Source: CAD feature listing. Evaluate the final solid. Frame: model axes, mm. Face numbers are marked on the shaded views. A direction names the side the tool comes from. Coordinates: 2 decimals unless noted, no trailing zeros. Write each loop counter-clockwise with the first axis right and the second up, starting at its lowest first coordinate (ties: lowest second). Pieces come first, ordered by that corner, then holes. Notation, with made-up numbers: (-33.75, 37) -> (-24.75, 37) arc R6 cw to (-24.75, 48) -> close; hole circle Ø10 at (54.25, -8.5). An arc over 180 degrees is marked (long way). One line per item, written item: value. Start each with the question number.
1. Access query for the marked faces 1, 2 and 3. Directions: +Z, -Z, +X, -X, +Y, -Y. A direction counts if a zero-diameter tool reaches every point of the face in a straight line with its end or side. Return the directions, or none.
2. Section query A-A, the plane z = -38. Output: boundary loops of the cut face in (x, y).
3. Mould query, pull axis X, two halves, no side actions, for the marked faces 4, 5 and 6. Classes: released by +X, released by -X, zero draft, split by the parting line, or undercut.
4. Section query C-C, the plane x = -18.5. Output: boundary loops of the cut face in (y, z).
5. First-contact query: P1, Ø1.8, axis at x = -19, y = -1, coming from the +Z side. Flat tip, straight axial feed; report the tip coordinate or a pass-through.
6. Section query B-B, the plane y = -5. Output: boundary loops of the cut face in (x, z).
7. Line query: line 1 (X direction, y = -1, z = -4); line 2 (X direction, y = -0.25, z = -26); line 3 (X direction, y = 0, z = -25). Output: solid intervals per line, ascending.
8. Section query D-D, the plane z = -5.5. Output: boundary loops of the cut face in (x, y), and give its area (3 significant figures).
from build123d import *

# Parameters (mm, degrees)
SALIENTE_EXTRUIR1_DEPTH = 39
CROQUIS2_W              = 8.25
CROQUIS2_H              = 28
CROQUIS2_W_2            = 1.05
CORTAR_EXTRUIR1_DEPTH   = 7
SALIENTE_EXTRUIR4_DEPTH = 3
SALIENTE_EXTRUIR5_DEPTH = 3
CROQUIS4_R              = 2.1
CORTAR_EXTRUIR2_DEPTH   = 52.548520832


with BuildPart() as part:
    # Croquis1 → Saliente-Extruir1 (new body)
    with BuildSketch(Plane.XY):
        with BuildLine():
            Line((-22.1, 1), (-28.5, 1))
            Line((-28.5, 1), (-28.5, -8))
            Line((-28.5, -8), (28.5, -8))
            Line((28.5, -8), (28.5, 1))
            Line((28.5, 1), (20.2, 1))
            ThreePointArc((20.2, 1), (15.5, -3.7), (10.8, 1))
            Line((10.8, 1), (1.2, 1))
            ThreePointArc((1.2, 1), (-3.5, -3.7), (-8.2, 1))
            Line((-8.2, 1), (-14.9, 1))
            ThreePointArc((-14.9, 1), (-18.5, -2.6), (-22.1, 1))
        make_face()
    extrude(amount=-SALIENTE_EXTRUIR1_DEPTH)

    # Croquis2 → Cortar-Extruir1 (cut)
    with BuildSketch(Plane(origin=(0, 1, 0), x_dir=(1, 0, 0), z_dir=(0, 1, 0))):
        with Locations((-19.025, 17.5)):
            Rectangle(CROQUIS2_W, CROQUIS2_H)
        with Locations((-14.375, 17.5)):
            Rectangle(CROQUIS2_W_2, CROQUIS2_H)
    extrude(amount=-CORTAR_EXTRUIR1_DEPTH, mode=Mode.SUBTRACT)

    # Croquis3 → Saliente-Extruir4 (add)
    with BuildSketch(Plane(origin=(0, 0, -39), x_dir=(-1, 0, 0), z_dir=(0, 0, -1))):
        with BuildLine():
            Line((-28.5, 1), (-28.5, -8))
            Line((-28.5, -8), (13.5, -8))
            Line((13.5, -8), (13.5, 1))
            Line((13.5, 1), (5, 1))
            ThreePointArc((5, 1), (3.5, -0.5), (2, 1))
            Line((2, 1), (-14, 1))
            ThreePointArc((-14, 1), (-15.5, -0.5), (-17, 1))
            Line((-17, 1), (-28.5, 1))
        make_face()
    extrude(amount=SALIENTE_EXTRUIR4_DEPTH)

    # Croquis3_4 → Saliente-Extruir5 (add, symmetric)
    with BuildSketch(Plane(origin=(0, 0, -39), x_dir=(-1, 0, 0), z_dir=(0, 0, -1))):
        with BuildLine():
            Line((13.5, 1), (13.5, -8))
            Line((13.5, -8), (28.5, -8))
            Line((28.5, -8), (28.5, 1))
            Line((28.5, 1), (20.5, 1))
            ThreePointArc((20.5, 1), (18.5, -1), (16.5, 1))
            Line((16.5, 1), (13.5, 1))
        make_face()
    extrude(amount=SALIENTE_EXTRUIR5_DEPTH, both=True)

    # Croquis4 → Cortar-Extruir2 (cut, through all)
    with BuildSketch(Plane(origin=(0, 1, 0), x_dir=(1, 0, 0), z_dir=(0, 1, 0))):
        with Locations(Location((-24.5, 38, 0), (0, 0, 270))):
            Circle(CROQUIS4_R)
        with Locations(Location((24.5, 38, 0), (0, 0, 270))):
            Circle(CROQUIS4_R)
        with Locations(Location((24.5, 4, 0), (0, 0, 270))):
            Circle(CROQUIS4_R)
    extrude(amount=-CORTAR_EXTRUIR2_DEPTH, mode=Mode.SUBTRACT)


solid = part.part
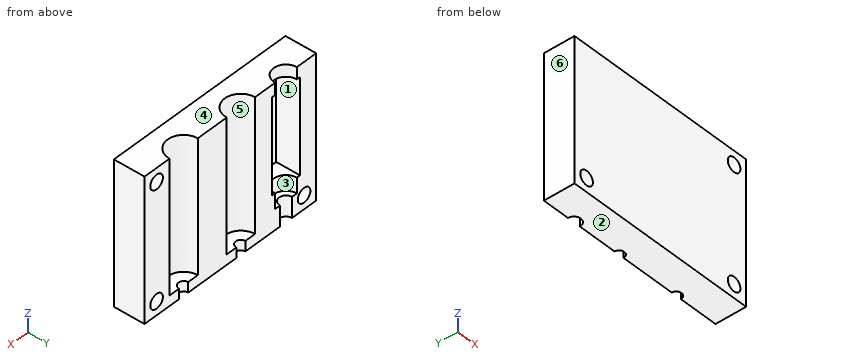
Computed values:
1. face 1: +Y
1. face 2: -Z, +X, -X, +Y, -Y
1. face 3: +Z, +Y
2. outline: (-28.5, -8) -> (-26.6, -8) -> (-26.6, 1) -> (-28.5, 1) -> close; (-22.4, -8) -> (22.4, -8) -> (22.4, 1) -> (20.2, 1) arc R4.7 cw to (10.8, 1) -> (1.2, 1) arc R4.7 cw to (-8.2, 1) -> (-16.5, 1) arc R2 cw to (-20.5, 1) -> (-22.4, 1) -> close; (26.6, -8) -> (28.5, -8) -> (28.5, 1) -> (26.6, 1) -> close
3. face 4: zero draft
3. face 5: undercut
3. face 6: released by -X
4. outline: (-8, -42) -> (-1, -42) -> (-1, -36) -> (-2.6, -36) -> (-2.6, -31.5) -> (-6, -31.5) -> (-6, -3.5) -> (-2.6, -3.5) -> (-2.6, 0) -> (-8, 0) -> close
5. P1: stops at z = -36
6. outline: (-28.5, -42) -> (28.5, -42) -> (28.5, 0) -> (-28.5, 0) -> close; hole circle Ø4.2 at (-24.5, -38); hole (-23.15, -31.5) -> (-13.85, -31.5) -> (-13.85, -3.5) -> (-23.15, -3.5) -> close; hole circle Ø4.2 at (24.5, -38); hole circle Ø4.2 at (24.5, -4)
7. line 1: x = -28.5 to -23.15, -13.85 to -7.75, 0.75 to 11.25, 19.75 to 22.4, 26.6 to 28.5
7. line 2: x = -28.5 to -23.15, -13.85 to -8.03, 1.03 to 10.97, 20.03 to 28.5
7. line 3: x = -28.5 to -23.15, -13.85 to -8.09, 1.09 to 10.91, 20.09 to 28.5
8. outline: (-28.5, -8) -> (23.03, -8) -> (23.03, 1) -> (20.2, 1) arc R4.7 cw to (10.8, 1) -> (1.2, 1) arc R4.7 cw to (-8.2, 1) -> (-13.85, 1) -> (-13.85, -6) -> (-23.15, -6) -> (-23.15, 1) -> (-28.5, 1) -> close; (25.97, -8) -> (28.5, -8) -> (28.5, 1) -> (25.97, 1) -> close
8. area: 352 mm²
